Solid Edge part; units mm, degrees
sketch "Sketch1" plane through (0, 0, 0) normal (0, 0, 1) x (1, 0, 0)
  line L0 (-34.3345, 10.1544) -> (-21.8345, 10.1544)
  line L1 (-21.8345, 10.1544) -> (-21.8345, 35.1544)
  line L2 (-21.8345, 35.1544) -> (-34.3345, 35.1544)
  line L3 (-34.3345, 35.1544) -> (-34.3345, 10.1544)
  dimension "D1" = 21.8345
  dimension "D2" = 34.3345
extrude "Protrusion1" add sketch "Sketch1" along normal blind 15.875
sketch "Sketch2" plane through (-28.0845, 22.6544, 0) normal (0, 0, -1) x (1, 0, 0)
  line L0 (-8.25, -14.5) -> (-8.25, 14.5)
  line L1 (-8.25, 14.5) -> (8.25, 14.5)
  line L2 (8.25, 14.5) -> (8.25, -14.5)
  line L3 (8.25, -14.5) -> (-8.25, -14.5)
extrude "ExtrudedProtrusion_2" add sketch "Sketch2" along normal blind 2
sketch "Sketch3" plane through (-28.0845, 22.6544, -2) normal (0, 0, -1) x (1, 0, 0)
  line L0 (-4.75, -11) -> (-4.75, 11)
  line L1 (-4.75, 11) -> (4.75, 11)
  line L2 (4.75, 11) -> (4.75, -11)
  line L3 (4.75, -11) -> (-4.75, -11)
extrude "ExtrudedProtrusion_3" add sketch "Sketch3" along normal blind 4
sketch "Sketch4" plane through (-32.8345, 22.6544, -4) normal (-1, 0, 0) x (0, 1, 0)
  line L0 (-11, 2) -> (0, 0.1136)
  line L1 (0, 0.1136) -> (11, 2)
extrude "Cutout1" cut sketch "Sketch4" against normal through all material side at (-32.8345, 17.1629, -5.1061)
fillet "Round_1" radius 0.5 7 edges at (-28.0845, 11.6544, -6) (-23.3345, 17.1544, -5.0568) (-28.0845, 22.6544, -4.1136) (-23.3345, 28.1544, -5.0568) (-28.0845, 33.6544, -6) (-32.8345, 28.1544, -5.0568) (-32.8345, 17.1544, -5.0568)
sketch "Sketch5" plane through (-28.0845, 22.6544, 15.875) normal (0, 0, 1) x (-1, 0, 0)
  line L0 (-3.2242, 0.4798) -> (3.7758, 0.4798)
  line L1 (3.7758, 0.4798) -> (3.7758, -0.5202)
  line L2 (3.7758, -0.5202) -> (-3.2242, -0.5202)
  line L3 (-3.2242, -0.5202) -> (-3.2242, 0.4798)
  line L4 (-3.2242, -7.7065) -> (3.7758, -7.7065)
  line L5 (3.7758, -7.7065) -> (3.7758, -8.7065)
  line L6 (3.7758, -8.7065) -> (-3.2242, -8.7065)
  line L7 (-3.2242, -8.7065) -> (-3.2242, -7.7065)
  line L8 (-3.2242, 9.5196) -> (3.7758, 9.5196)
  line L9 (3.7758, 9.5196) -> (3.7758, 8.5196)
  line L10 (3.7758, 8.5196) -> (-3.2242, 8.5196)
  line L11 (-3.2242, 8.5196) -> (-3.2242, 9.5196)
  dimension "D1" = 3.7758
  dimension "D2" = 3.2242
extrude "ExtrudedProtrusion_4" add sketch "Sketch5" along normal blind 10
sketch "Sketch6" plane through (-28.3603, 31.361, 20.875) normal (0, 1, 0) x (-1, 0, 0)
  line L0 (-4.074, 3.1687) -> (-1.2897, 5.953)
  line L1 (-1.2897, 5.953) -> (1.6313, 5.953)
  line L2 (1.6313, 5.953) -> (4.2278, 3.3737)
extrude "Cutout2" cut sketch "Sketch6" against normal through all material side at (-25.6431, 31.361, 25.4712)
sketch "Sketch7" plane through (-28.3603, 31.361, 20.875) normal (0, 1, 0) x (-1, 0, 0)
  circle A0 centre (0.174, 1.6484) radius 1.3058
extrude "Cutout3" cut sketch "Sketch7" against normal through all
sketch "Sketch8" plane through (-28.0845, 35.1544, 7.9375) normal (0, 1, 0) x (1, 0, 0)
  line L0 (0.9898, -7.9375) -> (-1.1525, -7.9375)
  line L1 (-1.1525, -7.9375) -> (-1.1525, 4.1896)
  line L2 (-1.1525, 4.1896) -> (0.9898, 4.1896)
  line L3 (0.9898, 4.1896) -> (0.9898, -7.9375)
extrude "ExtrudedProtrusion_5" add sketch "Sketch8" along normal blind 1
Here's how the part is built. I have some questions about the finished solid (model axes, mm). A direction names the side the tool comes from. Coordinates: 2 decimals unless noted, no trailing zeros. Order: outer loops, then holes, each group sorted by start corner. A loop starts at its lowest first (then second) coordinate and runs counter-clockwise, first axis right, second up. Notation, with made-up numbers: M -35.5,2.25 L -31.5,2.25 A28 cw -31.5,32.25 Z; hole C 34.5,61.25 d6. An arc over 180 degrees is marked long. Answer as CSV lines item,"result". Start each with the question number.
1. I want a section at B-B, the plane z = 22. Write out the boundary of the cut face in (x, y), and give its area (3 significant figures).
2. For pin 1 (4 mm diameter, centred on x = -25.5, y = 33.5, fed in from -Z); pin 2 (1.7 mm diameter, centred on x = -27.5, z = -4, fed in from -Y); pin 3 (0.5 mm diameter, centred on x = -28, y = 35.5, fed in from -Z); pin 4 (8 mm diameter, centred on y = 22, z = 9.5, fed in from -X), each with a flat end and sliding along its axis, tell me the tip position at first contact or that it passes through.
3. We'd pull the mould along X, two halves only. Please class faces 1 (the cylindrical face through (-29.137, 22.682, 21.365)), 2 (the flat face through (-28, 31.361, 21)), 3 (the flat face through (-31.4, 30.87, 25.43)), 4 (the flat face through (-19.834, 22, -1)): released by +X, released by -X, zero draft, split by the parting line, or undercut.
4. I need wall thicknesses on line 1 (Y direction, x = -27.75, z = 16.5); line 2 (X direction, y = 18, z = 8); line 3 (Z direction, x = -34.25, y = 27.25) (3 decimals). Which ranges of each line are inside material? Lowest first, please. Write a range as [from, to].
5. On a 3-axis mill with a long thin cutter (end or side, diameter ignored), from which of +Z, -Z, +X, -X, +Y, -Y can I reach the whole of each face in a straight line? I mean faces 5 (the flat face through (-28, 14.135, 21)), 6 (the cylindrical face through (-32.68, 28.25, -4.93)), 7 (the flat face through (-21.834, 22, 8)). Say none if no direction works.
6. I want a section at A-A, the plane z = 18. Write out the boundary of the cut face in (x, y), and give its area (3 significant figures).
7. I want a section at C-C, the plane x = -35. Write out the boundary of the cut face in (y, z).
8. I want a section at D-D, the plane z = 14.5. Write out the boundary of the cut face in (x, y).
Recorded:
1,outline,"M -31.86,13.13 L -29.73,13.13 L -29.73,14.13 L -31.86,14.13 Z; M -31.86,22.17 L -29.73,22.17 L -29.73,23.17 L -31.86,23.17 Z; M -31.86,30.36 L -29.73,30.36 L -29.73,31.36 L -31.86,31.36 Z; M -27.34,13.13 L -24.86,13.13 L -24.86,14.13 L -27.34,14.13 Z; M -27.34,22.17 L -24.86,22.17 L -24.86,23.17 L -27.34,23.17 Z; M -27.34,30.36 L -24.86,30.36 L -24.86,31.36 L -27.34,31.36 Z"
1,area,"13.8 mm2"
2,pin 1,"stops at z = -5.91"
2,pin 2,"stops at y = 11.65"
2,pin 3,"stops at z = -2"
2,pin 4,"stops at x = -34.33"
3,face 1,"undercut"
3,face 2,"zero draft"
3,face 3,"released by -X"
3,face 4,"released by +X"
4,line 1,"y = [13.13, 14.13], [22.17, 23.17], [30.36, 31.36]"
4,line 2,"x = [-34.33, -21.83]"
4,line 3,"z = [-2, 15.875]"
5,face 5,"+Z, +X, -X"
5,face 6,"-Z, -X"
5,face 7,"+Z, +X, +Y, -Y"
6,outline,"M -31.86,13.13 L -24.86,13.13 L -24.86,14.13 L -31.86,14.13 Z; M -31.86,22.17 L -24.86,22.17 L -24.86,23.17 L -31.86,23.17 Z; M -31.86,30.36 L -24.86,30.36 L -24.86,31.36 L -31.86,31.36 Z"
6,area,"21.0 mm2"
7,outline,"M 8.15,-2 L 37.15,-2 L 37.15,0 L 8.15,0 Z"
8,outline,"M -34.33,10.15 L -21.83,10.15 L -21.83,35.15 L -27.09,35.15 L -27.09,36.15 L -29.24,36.15 L -29.24,35.15 L -34.33,35.15 Z"
